Autodesk Inventor part; units mm, degrees
ref_plane "YZ Plane" through (0, 0, 0) normal (1, 0, 0) x (0, 1, 0)
ref_plane "XZ Plane" through (0, 0, 0) normal (0, 1, 0) x (-1, 0, 0)
ref_plane "XY Plane" through (0, 0, 0) normal (0, 0, 1) x (1, 0, 0)
sketch "Sketch1" plane through (0, 0, 0) normal (0, 0, 1) x (1, 0, 0)
  line L0 (0, 0) -> (50.8, 0)
  line L1 (50.8, 0) -> (50.8, 190.5)
  line L2 (50.8, 190.5) -> (0, 190.5)
  line L3 (0, 190.5) -> (0, 0)
  dimension "d0" = 50.8
  dimension "d1" = 190.5
extrude "Extrusion1" add sketch "Sketch1" along normal blind 6.35
sketch "Sketch2" plane through (0, 0, 6.35) normal (0, 0, 1) x (1, 0, 0)
  circle A0 centre (36.0934, 152.4) radius 7.9375
  line L0 (0, 0) -> (50.8, 0)
  line L1 (50.8, 0) -> (50.8, 190.5)
  dimension "d4" = 152.4
  dimension "d5" = 15.875
  dimension "d15" = 14.7066
extrude "Extrusion2" cut sketch "Sketch2" against normal blind 6.35
sketch "Sketch3" plane through (0, 0, 6.35) normal (0, 0, 1) x (1, 0, 0)
  line L0 (0, 190.5) -> (0, 0)
  line L1 (50.8, 0) -> (50.8, 190.5)
  line L2 (0, 177.8) -> (50.8, 177.8)
  line L3 (50.8, 177.8) -> (50.8, 190.5)
  line L4 (50.8, 190.5) -> (0, 190.5)
  line L5 (0, 190.5) -> (0, 177.8)
  dimension "d8" = 12.7
extrude "Extrusion3" cut sketch "Sketch3" against normal blind 25.4
sketch "Sketch4" plane through (0, 0, 6.35) normal (0, 0, 1) x (1, 0, 0)
  line L0 (0, 0) -> (50.8, 0)
  line L1 (0, 0) -> (-10.6807, 0)
  line L2 (-10.6807, 0) -> (-10.6807, 177.8)
  line L3 (-10.6807, 177.8) -> (0, 177.8)
  line L4 (0, 177.8) -> (0, 0)
  line L5 (50.8, 0) -> (61.4807, 0)
  line L6 (61.4807, 0) -> (61.4807, 177.8)
  line L7 (61.4807, 177.8) -> (50.8, 177.8)
  line L8 (50.8, 177.8) -> (50.8, 0)
  dimension "d11" = 10.6807
  dimension "d12" = 10.6807
extrude "Extrusion4" add sketch "Sketch4" against normal blind 6.35
properties part number "polycarb wall for saw blade"
Here's how the part is built. I have some questions about the finished solid (model axes, mm). Round coordinates to 2 decimals unless told otherwise and drop trailing zeros. Loops run counter-clockwise (first coordinate to the right, second up) from the corner with the lowest first, then second, coordinate; pieces in that order, holes last. Notation, with made-up numbers: M 46,-34 L 65,-34 A29 ccw 65,1 Z; hole C 47,52.25 d4. An arc over 180 degrees is marked long. Write each question's results on one line, items separated by ' | '. Start each with the question number.
(1) I want a section at A-A (y = 152.4). Please give me the cut outline in (x, z).
(2) I want a section at B-B (z = 1.75). Please give me the cut outline in (x, y) (1 decimal), then the cut area to 3 significant figures.
(3) If I drill on probe 1 along Y at (x, z) = (40, 5.5), over which ranges is the centre line in solid material (lowest first)? Write a range as from..to.
(4) Will this pin go through, and if not, where does the flat tip stop? P1, Ø10, axis at x = 10, y = 121.5, coming from the -Z side.
(5) Thinking about a two-plate mould opening in X: for faces 1 (the cylindrical face through (30.24, 157.76, 3.22)), 2 (the flat face through (-10.681, 88, 3)), 3 (the flat face through (25, 90, 6.35)), 4 (the flat face through (61.481, 88, 3)), which applies, pulls with the +X half, pulls with the -X half, needs draft (parallel to the pull), parting line crosses it, or undercut?
Solved:
1) outline: M -10.68,0 L 28.16,0 L 28.16,6.35 L -10.68,6.35 Z; M 44.03,0 L 61.48,0 L 61.48,6.35 L 44.03,6.35 Z
2) outline: M -10.7,0 L 61.5,0 L 61.5,177.8 L -10.7,177.8 Z; hole C 36.1,152.4 d15.9 | area: 12,600 mm²
3) probe 1: y = 0..145.49, 159.31..177.8
4) P1: stops at z = 0
5) face 1: undercut | face 2: pulls with the -X half | face 3: needs draft | face 4: pulls with the +X half
